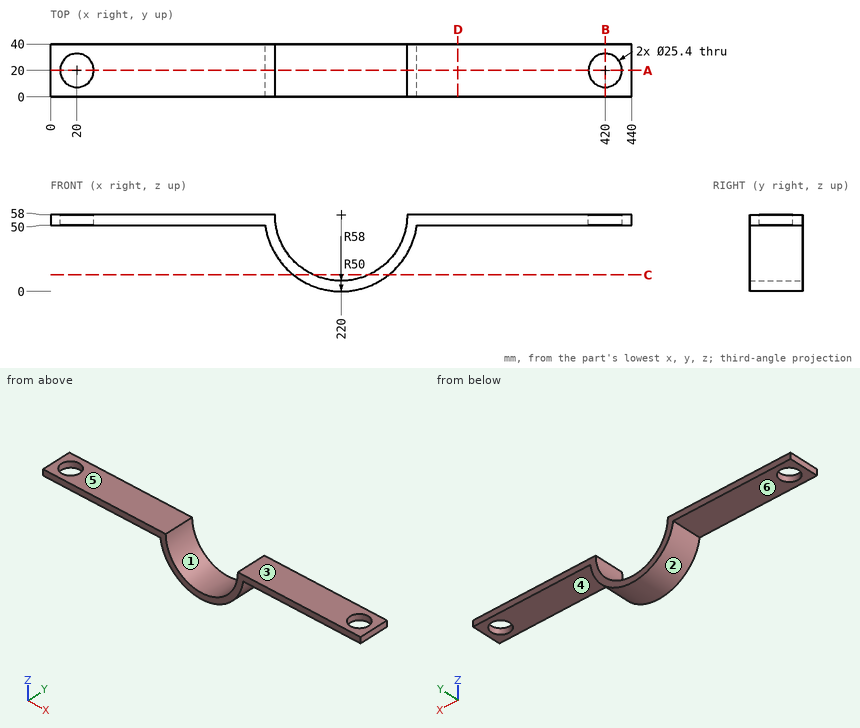
Check sheet for the drawn part. Datum: minimum x, y, z corner. Units: mm. A direction names the side the tool comes from. Round coordinates to 2 decimals unless told otherwise and drop trailing zeros. Loops run counter-clockwise (first coordinate to the right, second up) from the corner with the lowest first, then second, coordinate; pieces in that order, holes last. Notation, with made-up numbers: (-6.75, 56.5) -> (28.25, 56.5) arc R4 ccw to (28.25, 62.5) -> close; hole circle Ø11 at (79.5, 74). An arc over 180 degrees is marked (long way). Put each result on its own line as item: value. Start each with the question number.
1. Access from +Z, -Z, +X, -X, +Y, -Y to the whole of each face (thin tool, end or side, straight path). Record for the marked faces 4, 5 and 6.
2. Section check A-A (y = 20). Enter the section's corners in (x, z), plus the area to 3 significant figures.
3. Section check B-B (x = 420). Enter the section's corners in (y, z), plus the area to 3 significant figures.
4. Gauge pin test, flat ends, axial feed: pin 1 (3 mm diameter, centred on x = 194.5, y = 9, fed in from +Z); pin 2 (3 mm diameter, centred on x = 248.5, y = 8, fed in from +Z); pin 3 (2 mm diameter, centred on y = 33.5, z = 19, fed in from +X); pin 4 (10 mm diameter, centred on y = 12.5, z = 47, fed in from -X). Record the tip position at first contact, or that the pin passes through.
5. Section check D-D (x = 308.5). Enter the section's corners in (y, z).
6. Scan lines: probe 1 along Y at (x, z) = (420, 52.75); probe 2 along Z at (x, y) = (43.5, 25); probe 3 along X at (y, z) = (30.5, 34). Record each from-to range of solid material in increasing order.
7. Section check C-C (z = 12.5). Enter the section's corners in (x, y), plus the area to 3 significant figures.
8. Draft check along X on the marked faces 1, 2 and 3. Enter one of: +X half, -X half, draft (parallel to the pull), parting line (faces both ways), or undercut.
Findings:
1. face 4: -Z, +X, +Y, -Y
1. face 5: +Z, +X, -X, +Y, -Y
1. face 6: -Z, -X, +Y, -Y
2. outline: (0, 50) -> (7.3, 50) -> (7.3, 58) -> (0, 58) -> close; (32.7, 50) -> (162.55, 50) arc R58 ccw to (277.45, 50) -> (407.3, 50) -> (407.3, 58) -> (270, 58) arc R50 cw to (170, 58) -> (32.7, 58) -> close; (432.7, 50) -> (440, 50) -> (440, 58) -> (432.7, 58) -> close
2. area: 3,550 mm^2
3. outline: (0, 50) -> (7.3, 50) -> (7.3, 58) -> (0, 58) -> close; (32.7, 50) -> (40, 50) -> (40, 58) -> (32.7, 58) -> close
3. area: 117 mm^2
4. pin 1: stops at z = 15.92
4. pin 2: stops at z = 18
4. pin 3: stops at x = 263.82
4. pin 4: stops at x = 0
5. outline: (0, 50) -> (40, 50) -> (40, 58) -> (0, 58) -> close
6. probe 1: y = 0 to 7.3, 32.7 to 40
6. probe 2: z = 50 to 58
6. probe 3: x = 167.2 to 176.14, 263.86 to 272.8
7. outline: (184.03, 0) -> (199.27, 0) -> (199.27, 40) -> (184.03, 40) -> close; (240.73, 0) -> (255.97, 0) -> (255.97, 40) -> (240.73, 40) -> close
7. area: 1,220 mm^2
8. face 1: undercut
8. face 2: parting line
8. face 3: draft
